from build123d import *

# Parameters (mm, degrees)
SKETCH1_W           = 53.6
SKETCH1_H           = 39.6
BOSS_EXTRUDE1_DEPTH = 2
SKETCH2_W           = 53.6
SKETCH2_H           = 39.6
SKETCH2_W_2         = 49.6
SKETCH2_H_2         = 35.6
BOSS_EXTRUDE2_DEPTH = 20
SKETCH3_W           = 70
SKETCH3_H           = 60
SKETCH3_W_2         = 49.6
SKETCH3_H_2         = 35.6
BOSS_EXTRUDE3_DEPTH = 3
FILLET1_R           = 3


with BuildPart() as part:
    # Sketch1 → Boss-Extrude1 (new body)
    with BuildSketch(Plane(origin=(0, 0, 0), x_dir=(1, 0, 0), z_dir=(0, 1, 0))):
        Rectangle(SKETCH1_W, SKETCH1_H)
    extrude(amount=BOSS_EXTRUDE1_DEPTH)

    # Sketch2 → Boss-Extrude2 (add)
    with BuildSketch(Plane(origin=(0, 2, 0), x_dir=(1, 0, 0), z_dir=(0, 1, 0))):
        Rectangle(SKETCH2_W, SKETCH2_H)
        Rectangle(SKETCH2_W_2, SKETCH2_H_2, mode=Mode.SUBTRACT)
    extrude(amount=BOSS_EXTRUDE2_DEPTH)

    # Sketch3 → Boss-Extrude3 (add)
    with BuildSketch(Plane(origin=(0, 22, 0), x_dir=(1, 0, 0), z_dir=(0, 1, 0))):
        Rectangle(SKETCH3_W, SKETCH3_H)
        Rectangle(SKETCH3_W_2, SKETCH3_H_2, mode=Mode.SUBTRACT)
    extrude(amount=BOSS_EXTRUDE3_DEPTH)

    # Fillet1
    fillet1_edges = [part.edges().sort_by_distance(p)[0] for p in [
        (24.8, 13.5, 17.8),
        (0, 25, 17.8),
        (-24.8, 13.5, 17.8),
        (0, 2, 17.8),
        (24.8, 13.5, -17.8),
        (-24.8, 13.5, -17.8),
        (24.8, 2, 0),
        (-24.8, 2, 0),
        (0, 2, -17.8),
        (24.8, 25, 0),
        (0, 25, -17.8),
        (-24.8, 25, 0),
        (0, 25, 30),
        (0, 25, -30),
        (35, 25, 0),
        (-35, 25, 0),
    ]]
    fillet(fillet1_edges, radius=FILLET1_R - 0.0001)  # a hair under: the kernel refuses the full size


solid = part.part
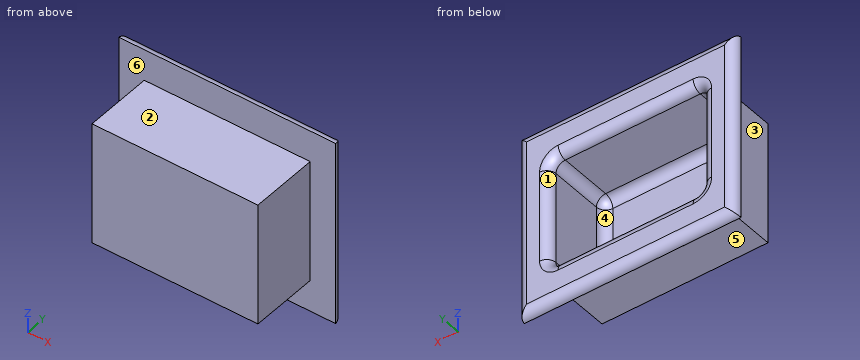
Work out the finished part from the listing and answer in its coordinate system (mm). Face numbers are marked on the shaded views. A direction names the side the tool comes from. Coordinates: 2 decimals unless noted, no trailing zeros. Write each loop counter-clockwise with the first axis right and the second up, starting at its lowest first coordinate (ties: lowest second). Pieces come first, ordered by that corner, then holes. Notation, with made-up numbers: M -36,84 L -8,84 A14 cw -8,100 Z; hole C 39,76 d8. An arc over 180 degrees is marked long. Use one line per item in the form item = value. Start each with the question number.
1. The mould has two halves that part along Z. Classify the marked faces 4, 5 and 6: released by +Z, released by -Z, zero draft, split by the parting line, or undercut.
2. The part is cut by section A-A (y = 13.75). Give the vertices of the cut face in (x, z), plus the area to 3 significant figures.
3. Straight lines are drawn through the part: probe 1 along Z at (x, y) = (7, 7.5); probe 2 along X at (y, z) = (6.5, -4); probe 3 along Y at (x, z) = (-30.5, -2.5). For each, find the intervals that lie inside material, in ascending order. Write a range as from..to.
4. A tool of negligible diameter and unlimited length cuts with its end or side. For the marked faces 1, 2 and 3, from which of +Z, -Z, +X, -X, +Y, -Y can it reach the whole face along a straight path? Write none if from no direction.
5. Each of these flat-tipped pins is pushed along its axis until it touches: P1, Ø1, axis at y = 21, z = -6.5, coming from the +X side; P2, Ø2, axis at x = -15, y = 11.5, coming from the +Z side; P3, Ø8, axis at y = 13, z = 0, coming from the -X side. Where does it stop, or does it pass through?
Evaluation:
q1.face_4 = undercut
q1.face_5 = released by -Z
q1.face_6 = zero draft
q2.outline = M -26.8,-19.8 L 26.8,-19.8 L 26.8,19.8 L -26.8,19.8 Z; hole M -24.8,-14.8 A3 ccw -21.8,-17.8 L 21.8,-17.8 A3 ccw 24.8,-14.8 L 24.8,14.8 A3 ccw 21.8,17.8 L -21.8,17.8 A3 ccw -24.8,14.8 Z
q2.area = 365 mm^2
q3.probe_1 = -19.8..-17.8, 17.8..19.8
q3.probe_2 = -26.8..-24.8, 24.8..26.8
q3.probe_3 = 22..25
q4.face_1 = +Y
q4.face_2 = +Z, +X, -X, -Y
q4.face_3 = +Z, -Z, -X, -Y
q5.P1 = 26.8
q5.P2 = 19.8
q5.P3 = -26.8
